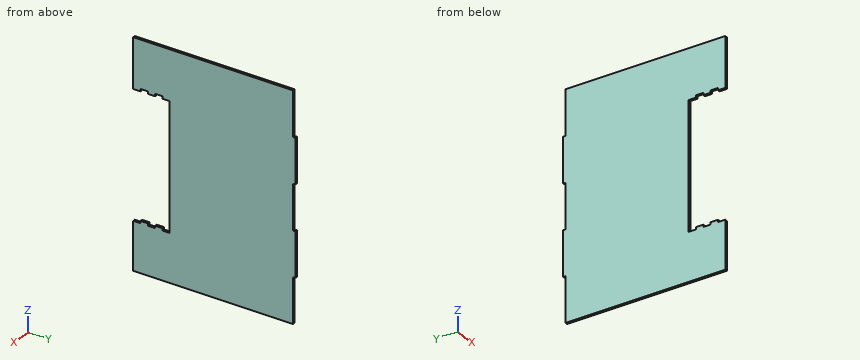
from build123d import *

# Parameters (mm, degrees)
BOSS_EXTRUDE1_DEPTH = 5


with BuildPart() as part:
    # Sketch1 → Boss-Extrude1 (new body)
    with BuildSketch(Plane(origin=(0, 0, 0), x_dir=(0, 0, -1), z_dir=(1, 0, 0))):
        Polygon((-247, 277.5), (-148.2, 277.5), (-148.2, 282.5), (-49.4, 282.5), (-49.4, 277.5), (49.4, 277.5), (49.4, 282.5), (148.2, 282.5), (148.2, 277.5), (247, 277.5), (247, -72.5), (141.262721236, -72.5), (141.262721236, -56.5), (136.262721236, -56.5), (136.262721236, -40.5), (141.262721236, -40.5), (141.262721236, -24.5), (136.262721236, -24.5), (136.262721236, -8.5), (141.262721236, -8.5), (141.262721236, 7.5), (0, 7.5), (-137.5, 7.5), (-137.5, -8.5), (-142.5, -8.5), (-142.5, -24.5), (-137.5, -24.5), (-137.5, -40.359311741), (-142.5, -40.5), (-142.5, -56.5), (-137.5, -56.5), (-137.5, -72.5), (-247, -72.5), align=None)
    extrude(amount=BOSS_EXTRUDE1_DEPTH)


solid = part.part
Read the model definition and answer for the solid it produces. Units are mm, in the model's axes. Give positions to 0.01 mm unless a question says otherwise; leave off trailing zeros. Write each loop counter-clockwise with the first axis right and the second up, starting at its lowest first coordinate (ties: lowest second). Pieces come first, ordered by that corner, then holes. Notation, with made-up numbers: (32, 18) - (80, 18) arc R28 cw to (80, 41) - close; hole circle Ø5 at (46.5, 40). An arc over 180 degrees is marked (long way). Answer in a Markdown table with one row per item. Add a question column.
Item 1: Section B-B, the plane z = -68.5 is taken. Write down the section's boundary in (x, y), and give its area (4 significant figures).
Item 2: Find the intervals of material crossed by L1, parallel to Y at x = 4.5, z = -78.5; L2, parallel to Y at x = 1.5, z = -154; L3, parallel to Z at x = 2.2, y = -54.5, in increasing order.
Item 3: Flat-ended cylindrical pins translate along their axes: P1, Ø1.5, axis at x = 3.5, z = -65.5, coming from the -Y side; P2, Ø1.5, axis at x = 3, z = -139.5, coming from the -Y side; P3, Ø1.5, axis at x = 3.5, z = 194.5, coming from the +Y side. Find the tip coordinate at first contact, or state that the pin passes through.
Item 4: Section C-C, the plane z = 11 is taken. Write down the section's boundary in (x, y).
Recorded:
| question | item | result |
|---|---|---|
| 1 | outline | (0, 7.5) - (5, 7.5) - (5, 282.5) - (0, 282.5) - close |
| 1 | area | 1,375 mm2 |
| 2 | L1 | y = 7.5 to 282.5 |
| 2 | L2 | y = -72.5 to 277.5 |
| 2 | L3 | z = -247 to -136.26, 142.5 to 247 |
| 3 | P1 | stops at y = 7.5 |
| 3 | P2 | stops at y = -56.5 |
| 3 | P3 | stops at y = 277.5 |
| 4 | outline | (0, 7.5) - (5, 7.5) - (5, 277.5) - (0, 277.5) - close |
